```python
from build123d import *

# Parameters (mm, degrees)
EXTRUDE_1_DEPTH     = 4
SKETCH_11_W         = 156
SKETCH_11_H         = 90
EXTRUDE_2_DEPTH     = 20
SKETCH_12_W         = 38
SKETCH_12_H         = 4
SKETCH_14_W         = 38
SKETCH_14_H         = 50
EXTRUDE_3_DEPTH     = 20
SKETCH_16_W         = 238.183586275
SKETCH_16_H         = 132.295328182
CUT_EXTRUDE_1_DEPTH = 10
SKETCH_17_W         = 40
SKETCH_17_H         = 20
EXTRUDE_4_DEPTH     = 4
SKETCH_21_R         = 6
SKETCH_21_R_2       = 4
EXTRUDE_8_DEPTH     = 4
EXTRUDE_11_DEPTH    = 15
EXTRUDE_12_DEPTH    = 8


with BuildPart() as part:
    # 草图1 → 凸台-拉伸1 (new body)
    with BuildSketch(Plane.XY):
        Polygon((-40, 0), (40, 0), (40, -160), (78, -160), (78, 0), (78, 50), (118, 90), (80, 90), (40, 50), (-40, 50), (-80, 90), (-118, 90), (-78, 50), (-78, 0), (-78, -160), (-40, -160), align=None)
    extrude(amount=EXTRUDE_1_DEPTH)

    # 草图11 → 凸台-拉伸2 (add)
    with BuildSketch(Plane.XY.offset(4)):
        with Locations((0, 5)):
            Rectangle(SKETCH_11_W, SKETCH_11_H)
    extrude(amount=EXTRUDE_2_DEPTH)

    # 扫描1: sweep along a path in 草图13
    with BuildLine(Plane(origin=(78, 0, 0), x_dir=(0, 0, -1), z_dir=(1, 0, 0))) as sweep_1_path:
        Line((-4, 90), (-4, 150))
        Line((-4, 150), (41, 227.942286341))
        Line((41, 227.942286341), (131, 227.942286341))
    # 草图12 → 扫描1 (sweep)
    with BuildSketch(Plane(origin=(0, 90, 0), x_dir=(1, 0, 0), z_dir=(0, 1, 0))):
        with Locations((-99, -2)):
            Rectangle(SKETCH_12_W, SKETCH_12_H)
        with Locations((99, -2)):
            Rectangle(SKETCH_12_W, SKETCH_12_H)
    sweep(path=sweep_1_path.line, transition=Transition.RIGHT)

    # 草图14 → 凸台-拉伸3 (add)
    with BuildSketch(Plane(origin=(0, 227.942286341, 0), x_dir=(1, 0, 0), z_dir=(0, 1, 0))):
        with Locations((-99, 106)):
            Rectangle(SKETCH_14_W, SKETCH_14_H)
        with Locations((99, 106)):
            Rectangle(SKETCH_14_W, SKETCH_14_H)
    extrude(amount=EXTRUDE_3_DEPTH)

    # 草图16 → 切除-拉伸1 (cut)
    with BuildSketch(Plane(origin=(0, 0, 0), x_dir=(-1, 0, 0), z_dir=(0, 0, -1))):
        with Locations((8.714033644, -106.147664091)):
            Rectangle(SKETCH_16_W, SKETCH_16_H)
    extrude(amount=-CUT_EXTRUDE_1_DEPTH, mode=Mode.SUBTRACT)

    # 草图17 → 凸台-拉伸4 (add)
    with BuildSketch(Plane.XZ.offset(40)):
        with Locations((0, 10)):
            Rectangle(SKETCH_17_W, SKETCH_17_H)
    extrude(amount=EXTRUDE_4_DEPTH)

    # 草图21 → 凸台-拉伸8 (add)
    with BuildSketch(Plane.XZ.offset(44)):
        with Locations((0, 9.5)):
            Circle(SKETCH_21_R)
        with Locations((0, 9.5)):
            Circle(SKETCH_21_R_2, mode=Mode.SUBTRACT)
    extrude(amount=EXTRUDE_8_DEPTH)

    # 草图28 → 凸台-拉伸11 (add, symmetric)
    with BuildSketch(Plane(origin=(0, 50, 0), x_dir=(1, 0, 0), z_dir=(0, 1, 0))):
        with BuildLine():
            Line((-122, 40), (-122, 97))
            Line((-122, 97), (-118, 97))
            Line((-118, 97), (-118, 40))
            ThreePointArc((-118, 40), (-106.284271247, 11.715728753), (-78, 0))
            Line((-78, 0), (-78, -4))
            ThreePointArc((-78, -4), (-109.112698372, 8.887301628), (-122, 40))
        make_face()
        with BuildLine():
            Line((118, 40), (118, 97))
            Line((118, 97), (122, 97))
            Line((122, 97), (122, 40))
            ThreePointArc((122, 40), (109.112698372, 8.887301628), (78, -4))
            Line((78, -4), (78, 0))
            ThreePointArc((78, 0), (106.284271247, 11.715728753), (118, 40))
        make_face()
    extrude(amount=EXTRUDE_11_DEPTH, both=True)

    # 草图29 → 凸台-拉伸12 (add)
    with BuildSketch(Plane(origin=(0, 50, 0), x_dir=(1, 0, 0), z_dir=(0, 1, 0))):
        Polygon((122, 97), (148, 97), (122, 71), align=None)
        Polygon((-122, 97), (-148, 97), (-122, 71), align=None)
    extrude(amount=-EXTRUDE_12_DEPTH)


solid = part.part
```
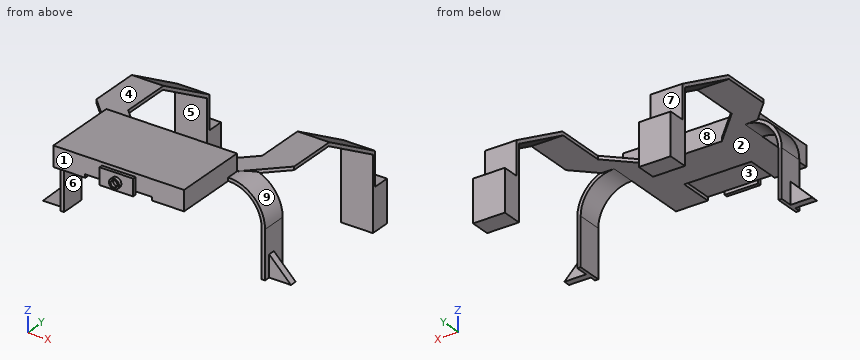
Could you check a few things on this model? Use its own coordinates, in mm. Face numbers are marked on the shaded views. A direction names the side the tool comes from. Round coordinates to 2 decimals unless told otherwise and drop trailing zeros. Loops run counter-clockwise (first coordinate to the right, second up) from the corner with the lowest first, then second, coordinate; pieces in that order, holes last. Notation, with made-up numbers: M 69,66.25 L 126,66.25 A21 ccw 126,81.25 Z; hole C 76.25,-31 d1. An arc over 180 degrees is marked long. Put each result on its own line as item: value.
Q1. On a 3-axis mill with a long thin cutter (end or side, diameter ignored), from which of +Z, -Z, +X, -X, +Y, -Y can I reach the whole of each face in a straight line? I mean the marked faces 5, 6, 7, 8 and 9. Say none if no direction works.
Check result:
face 5: -Z, +X, -X, -Y
face 6: -Z, -Y
face 7: +Z, +X, -X, +Y
face 8: +Z, +Y
face 9: +Z, +X, -Y
Q2. For pin 1 (13 mm diameter, centred on x = 98, z = -32, fed in from -Y); pin 2 (16 mm diameter, centred on x = 96.5, y = 239, fed in from +Z); pin 3 (7 mm diameter, centred on x = 34.5, z = 12, fed in from +Y), each with a flat end and sliding along its axis, tell me the tip position at first contact or that it passes through.
Check result:
pin 1: y = 193.1
pin 2: z = -81
pin 3: y = 50
Q3. Imagine slicing it at C-C (x = 0). Write out the boundary of the cut face in (y, z), then the cut area to 3 significant figures.
Check result:
outline: M -48,3.5 L -44,3.5 L -44,0 L -40,0 L -40,4 L 0,4 L 0,0 L 50,0 L 50,24 L -40,24 L -40,20 L -44,20 L -44,15.5 L -48,15.5 L -48,13.5 L -44,13.5 L -44,5.5 L -48,5.5 Z
area: 2,100 mm2
Q4. I need wall thicknesses on probe 1 along Z at (x, y) = (0, -45.95); probe 2 along Y at (x, z) = (125, -83); probe 3 along Y at (x, z) = (-115.5, -101). Which ranges of each line are inside material? Lowest first, please.
Check result:
probe 1: 3.5 to 5.5, 13.5 to 15.5
probe 2: 42 to 50
probe 3: 223.94 to 247.94
Q5. Imagine slicing it at B-B (z = -25). Write out the boundary of the cut face in (x, y).
Check result:
outline: M -119.36,35 L -115.08,35 L -115.08,65 L -119.36,65 Z; M -118,192.23 L -80,192.23 L -80,200.23 L -118,200.23 Z; M 80,192.23 L 118,192.23 L 118,200.23 L 80,200.23 Z; M 115.08,35 L 119.36,35 L 119.36,65 L 115.08,65 Z
Q6. Thinking about a two-plate mould opening in Y: for the marked faces 1, 2, 3 and 4, which applies, released by +Y, released by -Y, zero draft, split by the parting line, or undercut?
Check result:
face 1: released by -Y
face 2: undercut
face 3: undercut
face 4: zero draft
Q7. Imagine slicing it at A-A (y = 82). Write out the boundary of the cut face in (x, z), then the cut area to 3 significant figures.
Check result:
outline: M -110,0 L -72,0 L -72,4 L -110,4 Z; M 72,0 L 110,0 L 110,4 L 72,4 Z
area: 304 mm2
Q8. Imagine slicing it at D-D (z = 9.5). Write out the boundary of the cut face in (x, y).
Check result:
outline: M -78,-40 L -20,-40 L -20,-44 L -6,-44 L -6,-48 L -4,-48 L -4,-44 L 4,-44 L 4,-48 L 6,-48 L 6,-44 L 20,-44 L 20,-40 L 78,-40 L 78,50 L -78,50 Z
